Verification items for the finished model (mm, model axes). Face numbers are marked on the shaded views. A direction names the side the tool comes from. Round coordinates to 2 decimals unless told otherwise and drop trailing zeros. Loops run counter-clockwise (first coordinate to the right, second up) from the corner with the lowest first, then second, coordinate; pieces in that order, holes last. Notation, with made-up numbers: M -18,55 L 21,55 A11 ccw 21,71 Z; hole C -12.5,67.5 d6. An arc over 180 degrees is marked long. Answer as CSV lines item,"result".
```python
from build123d import *

# Parameters (mm, degrees)
F1_DEPTH   = 13.3858
F2_R       = 5.08
F3_R       = 2.06375
F4_DEPTH   = 25.4
F5_R       = 4.7625
F6_DEPTH   = 1.27
F7_C1_SIZE = 0.79375
F7_C2_SIZE = 0.79375
F7_C3_SIZE = 0.79365
F7_C4_SIZE = 0.79375
F8_SIZE    = 0.254


# Not quite as in the source:
# - a fillet or chamfer is up to 0.001 mm smaller than in the source, because OpenCascade refuses the exact size


with BuildPart() as f1:
    # F0 (on Right) → F1 (new body)
    with BuildSketch(Plane.YZ):
        with BuildLine():
            Line((10.16, -22.9468941689), (10.16, 25.0825))
            Line((10.16, 25.0825), (3.302, 25.0825))
            Line((3.302, 25.0825), (3.302, 0))
            ThreePointArc((3.302, 0), (0, -3.302), (-3.302, 0))
            ThreePointArc((-3.302, 0), (-6.731, 8.8281140591), (-10.16, 0))
            ThreePointArc((-10.16, 0), (-9.2901189355, -4.1133064758), (-6.8294310701, -7.5222650352))
            Line((-6.8294310701, -7.5222650352), (10.16, -22.9468941689))
        make_face()
    extrude(amount=F1_DEPTH)

    # F2
    f2_edges = [f1.edges().sort_by_distance(p)[0] for p in [
        (6.6929, 10.16, -22.946894),
        (13.3858, 6.731, 25.0825),
        (0, 6.731, 25.0825),
    ]]
    fillet(f2_edges, radius=F2_R)

    # F3 (on face) → F4 (cut)
    with BuildSketch(Plane.XZ.offset(-3.302)):
        with Locations((6.6929, 15.875)):
            Circle(F3_R)
    extrude(amount=-F4_DEPTH, mode=Mode.SUBTRACT)

    # F5 (on face) → F6 (cut)
    with BuildSketch(Plane.XZ.offset(-3.302)):
        with Locations((6.6929, 15.875)):
            Circle(F5_R)
    extrude(amount=-F6_DEPTH, mode=Mode.SUBTRACT)

    # F7: chamfer of 0.79375 on 16 edges, made by hand

    # F7_c1
    f7_c1_edges = [f1.edges().sort_by_distance(p)[0] for p in [
        (6.6929, 10.16, 25.0825),
        (1.4878975516, 10.16, 23.5946024484),
        (11.8979024484, 10.16, 23.5946024484),
        (0, 10.16, 4.2645264578),
        (13.3858, 10.16, 4.2645264578),
        (0, 7.1366532379, -16.1185065522),
        (0, -2.5820733026, -11.3784223186),
        (0, -9.2901189355, -4.1133064758),
        (13.3858, 7.1366532379, -16.1185065522),
        (13.3858, -2.5820733026, -11.3784223186),
        (13.3858, -9.2901189355, -4.1133064758),
    ]]
    chamfer(f7_c1_edges, length=F7_C1_SIZE)

    # F7_c2
    f7_c2_edges = [f1.edges().sort_by_distance(p)[0] for p in [
        (6.6929, 3.302, 25.0825),
        (1.4878975516, 3.302, 23.5946024484),
        (11.8979024484, 3.302, 23.5946024484),
        (0, 3.302, 10.00125),
        (0, 0, -3.302),
        (13.3858, 3.302, 10.00125),
        (13.3858, 0, -3.302),
    ]]
    chamfer(f7_c2_edges, length=F7_C2_SIZE)

    # F7_c3 (size 0.79375 in the source; OpenCascade refuses exactly that, so slightly less here)
    f7_c3_edges = [f1.edges().sort_by_distance(p)[0] for p in [
        (0, -6.731, 8.8281140591),
    ]]
    chamfer(f7_c3_edges, length=F7_C3_SIZE)

    # F7_c4
    f7_c4_edges = [f1.edges().sort_by_distance(p)[0] for p in [
        (13.3858, -6.731, 8.8281140591),
    ]]
    chamfer(f7_c4_edges, length=F7_C4_SIZE)

    # F8
    f8_edges = [f1.edges().sort_by_distance(p)[0] for p in [
        (11.4554, 3.937, 15.875),
        (1.9304, 3.302, 15.875),
        (1.9304, 4.572, 15.875),
        (4.62915, 4.572, 15.875),
        (8.75665, 7.366, 15.875),
        (4.62915, 10.16, 15.875),
    ]]
    chamfer(f8_edges, length=F8_SIZE)


solid = f1.part
```
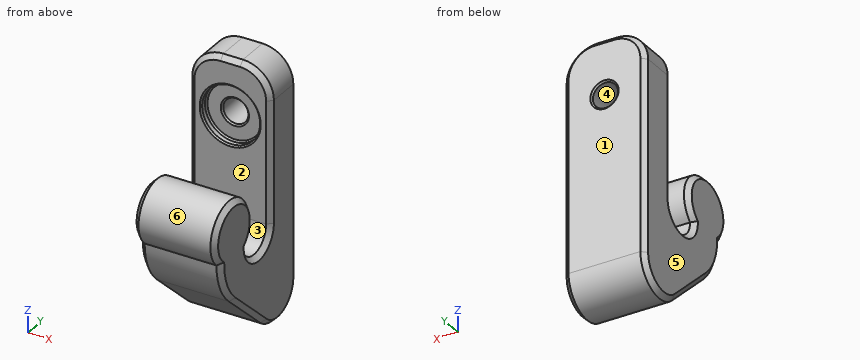
1) Section check A-A (y = 0). Record the cut outline in (x, z), plus the area to 3 significant figures.
Here are the results:
outline,"M 0,-12.65 L 0.79,-13.72 L 12.59,-13.72 L 13.39,-12.65 L 13.39,-4.1 L 12.59,-3.3 L 0.79,-3.3 L 0,-4.1 Z"
area,"138 mm^2"
2) Draft check along X on the marked faces 4, 5 and 6. Enter one of: +X half, -X half, draft (parallel to the pull), parting line (faces both ways), or undercut.
Here are the results:
face 4,"undercut"
face 5,"-X half"
face 6,"draft"
3) Material ranges on probe 1 along Z at (x, y) = (4.75, -2.25) (3 decimals); probe 2 along Y at (x, z) = (9.25, -2.5); probe 3 along Y at (x, z) = (11.75, 4.5), recorded low to high.
Here are the results:
probe 1,"z = -11.68 to -2.417, 1.355 to 6.141"
probe 2,"y = -9.85 to -2.16, 2.16 to 10.16"
probe 3,"y = -11.76 to -1.71, 3.3 to 10.16"
4) Go/stop test with flat-tipped pins: pin 1 (6 mm diameter, centred on x = 8.5, y = 4.5, fed in from +Z); pin 2 (8 mm diameter, centred on x = 9.5, y = -0.5, fed in from -Z); pin 3 (5.5 mm diameter, centred on x = 6.69, z = 15.88, fed in from -Y); pin 4 (8 mm diameter, centred on x = 10.5, y = -6, fed in from -Z). Record where each tip stops, or that it passes through.
Here are the results:
pin 1,"stops at z = 25.08"
pin 2,"stops at z = -16.3"
pin 3,"stops at y = 4.57"
pin 4,"stops at z = -11.91"
5) Set-up check for the marked faces 1, 2 and 3: record each of +Z, -Z, +X, -X, +Y, -Y from which the full face is reachable in a straight line by a thin tool's end or side.
Here are the results:
face 1,"+Z, -Z, +X, -X, +Y"
face 2,"+Z, +X, -X"
face 3,"+X, -X"
6) Section check B-B (z = -10.5). Record the cut outline in (x, y).
Here are the results:
outline,"M 0,-2.37 L 0.79,-3.55 L 12.59,-3.55 L 13.39,-2.37 L 13.39,9.37 L 12.59,10.16 L 0.79,10.16 L 0,9.37 Z"
